Verification items for the finished model (mm, model axes). Face numbers are marked on the shaded views. Coordinates: 2 decimals unless noted, no trailing zeros. Loops run counter-clockwise (first coordinate to the right, second up) from the corner with the lowest first, then second, coordinate; pieces in that order, holes last. Notation, with made-up numbers: M -7,29.5 L 38,29.5 A4 ccw 38,35.5 Z; hole C 52,18.5 d2. An arc over 180 degrees is marked long. Write item = value, one per line. Start each with the question number.
```python
from build123d import *

# Parameters (mm, degrees)
F1_DEPTH   = 180
F2_R       = 2
F3_DEPTH   = 25
F4_R       = 6
F4_R_2     = 2
F5_DEPTH   = 3
F6_W       = 14.0674761496
F6_H       = 116.9483624399
F1_FACE1_W = 20.2
F1_FACE1_H = 180
F1_FACE1_R = 6
F7_DEPTH   = 0.5
F9_DEPTH   = 25
F10_W      = 4.3
F10_H      = 12
F11_DEPTH  = 25
F12_W      = 4.3
F12_H      = 12
F13_DEPTH  = 25


with BuildPart() as f1:
    # F0 (on Front) → F1 (new body)
    with BuildSketch(Plane.XZ):
        Polygon((5.8, 4.7), (-5.8, 4.7), (-5.8, 0.5), (-10.1, 0.5), (-10.1, -4.7), (10.1, -4.7), (10.1, 0.5), (5.8, 0.5), align=None)
    extrude(amount=F1_DEPTH)

    # F2 (on face) → F3 (cut)
    with BuildSketch(Plane.XY.offset(4.7)):
        with Locations((0, -140)):
            Circle(F2_R)
        with Locations((0, -90)):
            Circle(F2_R)
        with Locations((-0.0078984785, -40.0161966681)):
            Circle(F2_R)
    extrude(amount=-F3_DEPTH, mode=Mode.SUBTRACT)

    # F4 (on face) → F5 (cut)
    with BuildSketch(Plane(origin=(0, 0, -4.7), x_dir=(1, 0, 0), z_dir=(0, 0, -1))):
        with Locations((-0.0078984785, 40.0161966681)):
            Circle(F4_R)
        with Locations((-0.0078984785, 40.0161966681)):
            Circle(F4_R_2, mode=Mode.SUBTRACT)
        with Locations((0, 90)):
            Circle(F4_R)
        with Locations((0, 90)):
            Circle(F4_R_2, mode=Mode.SUBTRACT)
        with Locations((0, 140)):
            Circle(F4_R)
        with Locations((0, 140)):
            Circle(F4_R_2, mode=Mode.SUBTRACT)
    extrude(amount=-F5_DEPTH, mode=Mode.SUBTRACT)

    # F6 (on face) + F1_face1 (on face) → F7 (join)
    with BuildSketch(Plane(origin=(0, 0, -1.7), x_dir=(1, 0, 0), z_dir=(0, 0, -1))):
        with Locations((0.141544966, 90.3544295579)):
            Rectangle(F6_W, F6_H)
    with BuildSketch(Plane(origin=(2.75839e-05, -89.9999434363, -4.7), x_dir=(1, 0, 0), z_dir=(0, 0, -1))):
        with Locations((-2.75839e-05, 5.65637e-05)):
            Rectangle(F1_FACE1_W, F1_FACE1_H)
        with Locations((-2.75839e-05, 50.0000565637)):
            Circle(F1_FACE1_R, mode=Mode.SUBTRACT)
        with Locations((-0.0079260625, -49.9837467681)):
            Circle(F1_FACE1_R, mode=Mode.SUBTRACT)
        with Locations((-2.75839e-05, 5.65637e-05)):
            Circle(F1_FACE1_R, mode=Mode.SUBTRACT)
    extrude(amount=F7_DEPTH)

    # F8 (on face) → F9 (cut)
    with BuildSketch(Plane.XY.offset(4.7)):
        Polygon((5.8, -180), (5.8, -168), (0, -180), align=None)
        Polygon((0, -180), (-5.8, -168), (-5.8, -180), align=None)
        Polygon((0, -12), (5.8, 0), (-5.8, 0), align=None)
    extrude(amount=-F9_DEPTH, mode=Mode.SUBTRACT)

    # F10 (on face) → F11 (cut)
    with BuildSketch(Plane.XY.offset(0.5)):
        with Locations((7.95, -174)):
            Rectangle(F10_W, F10_H)
    extrude(amount=-F11_DEPTH, mode=Mode.SUBTRACT)

    # F12 (on face) → F13 (cut)
    with BuildSketch(Plane.XY.offset(0.5)):
        with Locations((-7.95, -174)):
            Rectangle(F12_W, F12_H)
    extrude(amount=-F13_DEPTH, mode=Mode.SUBTRACT)


solid = f1.part
```
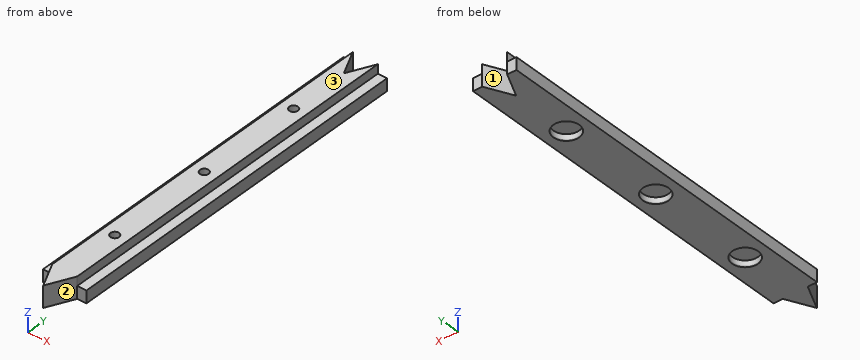
Q1. Mould release check, pull along X, two halves, no side actions. Record for the marked faces 1, 2 and 3: +X half, -X half, draft (parallel to the pull), parting line (faces both ways), or undercut.
Q2. Sectioned sample at B-B on z = 2.75. Record the cut outline in (x, y).
Q3. Sectioned sample at D-D on y = -43.5. Record the cut outline in (x, z).
Q4. Sectioned sample at C-C on x = -3.5. Record the cut outline in (y, z), plus the area to 3 significant figures.
Q5. Gauge pin test, flat ends, axial feed: pin 1 (7 mm diameter, centred on x = 0, y = -140, fed in from -Z); pin 2 (1.5 mm diameter, centred on x = 4, z = 2, fed in from -Y); pin 3 (2 mm diameter, centred on y = -105.5, z = 2, fed in from -X). Record the tip position at first contact, or that the pin passes through.
Q6. Scan lines: L1, parallel to X at y = -90, z = 3; L2, parallel to X at y = -90, z = -4.95; L3, parallel to Y at x = 0.5, z = 0.75. Record each from-to range of solid material in increasing order. Write a range as [from, to].
Q7. Sectioned sample at A-A on y = -101. Record the cut outline in (x, z), plus the area to 3 significant figures.
Solutions:
q1.face_1 = undercut
q1.face_2 = +X half
q1.face_3 = draft
q2.outline = M -5.8,-168 L 0,-180 L 5.8,-168 L 5.8,0 L 0,-12 L -5.8,0 Z; hole C -0.01,-40.02 d4; hole C 0,-140 d4; hole C 0,-90 d4
q3.outline = M -10.1,-5.2 L -4.89,-5.2 L -4.89,-2.2 L 4.88,-2.2 L 4.88,-5.2 L 10.1,-5.2 L 10.1,0.5 L 5.8,0.5 L 5.8,4.7 L -5.8,4.7 L -5.8,0.5 L -10.1,0.5 Z
q4.outline = M -172.76,-5.2 L -144.87,-5.2 L -144.87,-2.2 L -135.13,-2.2 L -135.13,-5.2 L -94.87,-5.2 L -94.87,-2.2 L -85.13,-2.2 L -85.13,-5.2 L -44.9,-5.2 L -44.9,-2.2 L -35.14,-2.2 L -35.14,-5.2 L -4.76,-5.2 L -4.76,4.7 L -172.76,4.7 Z
q4.area = 1,580 mm²
q5.pin_1 = -2.2
q5.pin_2 = -173.28
q5.pin_3 = -5.8
q6.L1 = [-5.8, -2], [2, 5.8]
q6.L2 = [-10.1, -6], [6, 10.1]
q6.L3 = [-178.97, -141.94], [-138.06, -91.94], [-88.06, -41.95], [-38.08, -10.97]
q7.outline = M -10.1,-5.2 L 10.1,-5.2 L 10.1,0.5 L 5.8,0.5 L 5.8,4.7 L -5.8,4.7 L -5.8,0.5 L -10.1,0.5 Z
q7.area = 164 mm²
